Input: part model. Units: mm. Frame: model coordinates. Face numbers are marked on the shaded views. A direction names the side the tool comes from. Give positions to 0.01 mm unless a question says otherwise; leave off trailing zeros. Write each loop counter-clockwise with the first axis right and the second up, starting at its lowest first coordinate (ties: lowest second). Pieces come first, ordered by that corner, then holes.
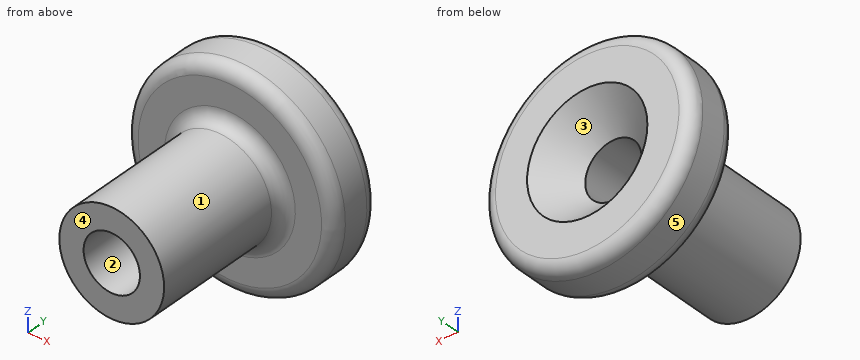
```python
from build123d import *

# Parameters (mm, degrees)
REDONDEO1_R                                          = 1
AVELLANADO_PARA_TORNILLO_CON_CABEZA_AVEL_D           = 4.3
AVELLANADO_PARA_TORNILLO_CON_CABEZA_AVEL_CSINK_D     = 9.18
AVELLANADO_PARA_TORNILLO_CON_CABEZA_AVEL_CSINK_ANGLE = 90


with BuildPart() as part:
    # Croquis1 → Revolución1 (revolve)
    with BuildSketch(Plane.XY, mode=Mode.PRIVATE) as revoluci_n1_sk:
        Polygon((0, 15), (8, 15), (8, 11), (4, 11), (4, 0), (0, 0), align=None)
    revolve(revoluci_n1_sk.sketch.rotate(Axis((0, 0, 0), (0, 1, 0)), 90), axis=Axis((0, 0, 0), (0, 1, 0)))

    # Redondeo1
    redondeo1_edges = [part.edges().sort_by_distance(p)[0] for p in [
        (0, 11, 4),
        (0, 11, 8),
        (0, 15, 8),
    ]]
    fillet(redondeo1_edges, radius=REDONDEO1_R)

    # Avellanado para tornillo con cabeza avellanada de clavija hexagonal de M41 (through all)
    with Locations(Plane(origin=(0, 15, 0), x_dir=(1, 0, 0), z_dir=(0, 1, 0))):
        with Locations((0, 0)):
            CounterSinkHole(AVELLANADO_PARA_TORNILLO_CON_CABEZA_AVEL_D / 2, AVELLANADO_PARA_TORNILLO_CON_CABEZA_AVEL_CSINK_D / 2, counter_sink_angle=AVELLANADO_PARA_TORNILLO_CON_CABEZA_AVEL_CSINK_ANGLE)


solid = part.part
```
Item 1: Mould query, pull axis X, two halves, no side actions, for the marked faces 3, 4 and 5. Classes: +X half, -X half, draft (parallel to the pull), parting line (faces both ways), or undercut.
Item 2: Section A-A (x = 0). Return loops of the section in (y, z), and give its area (3 significant figures).
Item 3: Pin query (flat end, axial travel): pin 1 (6 mm diameter, centred on x = -5.5, z = -6, fed in from -Y); pin 2 (1 mm diameter, centred on x = -6, y = 11.5, fed in from -Z). Return the tip coordinate at first contact, or that it passes through.
Item 4: Section C-C (y = 5.5). Return loops of the section in (x, z), and give its area (3 significant figures).
Item 5: Ray query, line 1 (Y direction, x = -7, z = -0.25); line 2 (X direction, y = 6.5, z = -1.75); line 3 (X direction, y = 14.75, z = -2). Return the intervals inside material, ascending.
Item 6: Set-up query: the marked faces 1 and 2. Return all of +Z, -Z, +X, -X, +Y, -Y with unobstructed straight access to the full face (end or side cutting, diameter ignored); none if empty.
Item 7: Section B-B (z = 0). Return loops of the section in (x, y), and give its area (3 significant figures).
Item 8: Section D-D (y = 11.25). Return loops of the section in (x, z).
Solved:
1. face 3: undercut
1. face 4: draft
1. face 5: parting line
2. outline: (0, -4) - (10, -4) arc R1 cw to (11, -5) - (11, -7) arc R1 ccw to (12, -8) - (14, -8) arc R1 ccw to (15, -7) - (15, -4.59) - (12.56, -2.15) - (0, -2.15) - close; (0, 2.15) - (12.56, 2.15) - (15, 4.59) - (15, 7) arc R1 ccw to (14, 8) - (12, 8) arc R1 ccw to (11, 7) - (11, 5) arc R1 cw to (10, 4) - (0, 4) - close
2. area: 81.1 mm2
3. pin 1: stops at y = 11
3. pin 2: stops at z = -5.71
4. outline: circle Ø8 at (0, 0); hole circle Ø4.3 at (0, 0)
4. area: 35.7 mm2
5. line 1: y = 11 to 15
5. line 2: x = -3.6 to -1.25, 1.25 to 3.6
5. line 3: x = -7.4 to -3.85, 3.85 to 7.4
6. face 1: -Y
6. face 2: +Y, -Y
7. outline: (-8, 12) arc R1 ccw to (-7, 11) - (-5, 11) arc R1 cw to (-4, 10) - (-4, 0) - (-2.15, 0) - (-2.15, 12.56) - (-4.59, 15) - (-7, 15) arc R1 ccw to (-8, 14) - close; (2.15, 0) - (4, 0) - (4, 10) arc R1 cw to (5, 11) - (7, 11) arc R1 ccw to (8, 12) - (8, 14) arc R1 ccw to (7, 15) - (4.59, 15) - (2.15, 12.56) - close
7. area: 81.1 mm2
8. outline: circle Ø15.32 at (0, 0); hole circle Ø4.3 at (0, 0)
